Geometry: see drawing. Coordinates: mm, zero at the bounding-box minimum. Coordinates: 2 decimals unless noted, no trailing zeros. Loops run counter-clockwise (first coordinate to the right, second up) from the corner with the lowest first, then second, coordinate; pieces in that order, holes last. Notation, with made-up numbers: (14, 7.25) -> (38, 7.25) arc R11 cw to (38, 11.25) -> close; hole circle Ø9 at (2.25, 1). An arc over 180 degrees is marked (long way). One line per question, with ' | ' between items. Start each with the question number.
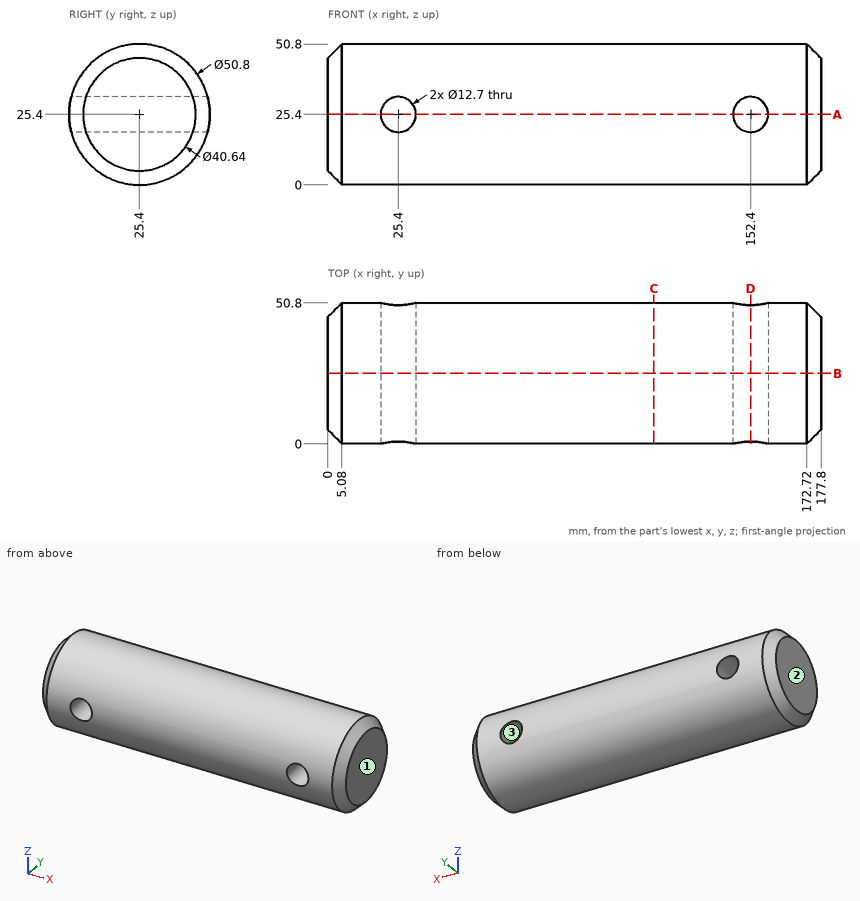
(1) Ray query, L1, parallel to X at y = 15, z = 25; L2, parallel to X at y = 7.5, z = 28.5; L3, parallel to Y at x = 56.5, z = 26.5. Return the intervals inside material, ascending.
(2) Cut plane A-A, the plane z = 25.4. Return the cut outline in (x, y).
(3) Cut plane D-D, the plane x = 152.4. Return the cut outline in (y, z), and give its area (3 significant figures).
(4) Cut plane C-C, the plane x = 117.5. Return the cut outline in (y, z).
(5) Cut plane B-B, the plane y = 25.4. Return the cut outline in (x, z), and give its area (3 significant figures).
(6) Contact query for flat-ended pins moving along their axis: pin 1 Ø6 at (x, z) = (75.5, 33.5) entering from +Y; pin 2 Ø10 at (x, y) = (47.5, 29) entering from +Z; pin 3 Ø1 at (x, z) = (160, 34) entering from -Y; pin 4 Ø7.5 at (x, z) = (152.4, 25.4) entering from -Y. Output: stop coordinate, or through.
(7) Draft query along X for the marked faces 1, 2 and 3. Return one class per face: pulls with the +X half, pulls with the -X half, needs draft (parallel to the pull), parting line crosses it, or undercut.
Here are the results:
1) L1: x = 0 to 19.06, 31.74 to 146.06, 158.74 to 177.8 | L2: x = 0 to 19.86, 30.94 to 146.86, 157.94 to 177.8 | L3: y = 0.02 to 50.78
2) outline: (0, 5.08) -> (5.08, 0) -> (19.05, 0) -> (19.05, 50.8) -> (5.08, 50.8) -> (0, 45.72) -> close; (31.75, 0) -> (146.05, 0) -> (146.05, 50.8) -> (31.75, 50.8) -> close; (158.75, 0) -> (172.72, 0) -> (177.8, 5.08) -> (177.8, 45.72) -> (172.72, 50.8) -> (158.75, 50.8) -> close
3) outline: (0.81, 19.05) arc R25.4 ccw to (49.99, 19.05) -> close; (0.81, 31.75) -> (49.99, 31.75) arc R25.4 ccw to start | area: 1,390 mm2
4) outline: circle Ø50.8 at (25.4, 25.4)
5) outline: (0, 5.08) -> (5.08, 0) -> (172.72, 0) -> (177.8, 5.08) -> (177.8, 45.72) -> (172.72, 50.8) -> (5.08, 50.8) -> (0, 45.72) -> close; hole circle Ø12.7 at (25.4, 25.4); hole circle Ø12.7 at (152.4, 25.4) | area: 8,730 mm2
6) pin 1: stops at y = 50.28 | pin 2: stops at z = 50.8 | pin 3: stops at y = 1.33 | pin 4: passes through
7) face 1: pulls with the +X half | face 2: pulls with the -X half | face 3: undercut
